from build123d import *

# Parameters (mm, degrees)
F1_DEPTH = 13
F2_R     = 1.5
F4_DEPTH = 4
F5_ANGLE = -90


with BuildPart() as f1:
    # F0 (on Top) → F1 (new body)
    with BuildSketch(Plane.XY):
        Polygon((-40, -45), (-45, 0), (0, 0), (45, 0), (40, -45), (45, -45), (50, 0), (50, 7), (45, 7), (44.8581193677, 7), (-44.8581193677, 7), (-45, 7), (-50, 7), (-50, 0), (-45, -45), align=None)
    extrude(amount=F1_DEPTH)

    # F2
    f2_edges = [f1.edges().sort_by_distance(p)[0] for p in [
        (-42.5, -22.5, 13),
        (0, 0, 13),
        (42.5, -22.5, 13),
        (42.5, -45, 13),
        (47.5, -22.5, 13),
        (50, 3.5, 13),
        (0, 7, 13),
        (-50, 3.5, 13),
        (-47.5, -22.5, 13),
        (-42.5, -45, 13),
        (-42.5, -22.5, 0),
        (0, 0, 0),
        (42.5, -22.5, 0),
        (42.5, -45, 0),
        (47.5, -22.5, 0),
        (50, 3.5, 0),
        (0, 7, 0),
        (-50, 3.5, 0),
        (-47.5, -22.5, 0),
        (-42.5, -45, 0),
        (40, -45, 6.5),
        (45, -45, 6.5),
        (-45, -45, 6.5),
        (-40, -45, 6.5),
        (-45, 0, 6.5),
        (45, 0, 6.5),
        (-50, 7, 6.5),
        (-50, 0, 6.5),
        (50, 0, 6.5),
        (50, 7, 6.5),
    ]]
    fillet(f2_edges, radius=F2_R)

    # F3 (on face) → F4 (cut)
    with BuildSketch(Plane.XZ):
        with BuildLine():
            Line((-14.1421356237, 2.9644660941), (-15.6066017178, 1.5))
            Line((-15.6066017178, 1.5), (15.6066017178, 1.5))
            Line((15.6066017178, 1.5), (14.1421356237, 2.9644660941))
            ThreePointArc((14.1421356237, 2.9644660941), (12.6776695297, 6.5), (14.1421356237, 10.0355339059))
            Line((14.1421356237, 10.0355339059), (15.6066017178, 11.5))
            Line((15.6066017178, 11.5), (-15.6066017178, 11.5))
            Line((-15.6066017178, 11.5), (-14.1421356237, 10.0355339059))
            ThreePointArc((-14.1421356237, 10.0355339059), (-12.6776695297, 6.5), (-14.1421356237, 2.9644660941))
        make_face()
        Polygon((-24.8033008589, 20.6966991411), (-15.6066017178, 11.5), (15.6066017178, 11.5), (24.8033008589, 20.6966991411), (19.5, 26), (14.1966991411, 31.3033008589), (0, 17.1066017178), (-14.1966991411, 31.3033008589), (-19.5, 26), align=None)
        Polygon((-24.8033008589, -7.6966991411), (-19.5, -13), (-14.1966991411, -18.3033008589), (0, -4.1066017178), (14.1966991411, -18.3033008589), (19.5, -13), (24.8033008589, -7.6966991411), (15.6066017178, 1.5), (-15.6066017178, 1.5), align=None)
    extrude(amount=-F4_DEPTH, mode=Mode.SUBTRACT)


with BuildPart() as f1_1:
    # F5: moved
    add(f1.part.rotate(Axis((0, 4, 0), (1, 0, 0)), F5_ANGLE))


solid = f1_1.part
Design review of the part built by this model. Coordinates are the model's own, in mm. A direction names the side the tool comes from. Give positions to 0.01 mm unless a question says otherwise; leave off trailing zeros. Order: outer loops, then holes, each group sorted by start corner. A loop starts at its lowest first (then second) coordinate and runs counter-clockwise, first axis right, second up.
1. Add section A-A, the plane x = -5. State the section outline as (y, z) points, then the cut area to 3 significant figures.
Solution:
outline: (4, -1.5) arc R1.5 ccw to (5.5, -3) - (15.5, -3) arc R1.5 ccw to (17, -1.5) - (17, 0) - (4, 0) - close
area: 38.0 mm2
2. Mouldability with a two-part tool opening along Z and no side actions: class faces 1 (the flat face through (0, 17, -1)), 2 (the flat face through (-42.468, 10.43, 26.792)), 3 (the flat face through (1, 10, -3)) as +Z half, -Z half, draft (parallel to the pull), parting line (faces both ways), or undercut.
Solution:
face 1: draft
face 2: undercut
face 3: -Z half
3. To check wall thickness, follow L1, parallel to Z at x = -17, y = 8.25; L2, parallel to Z at x = 6, y = 8.75; L3, parallel to X at y = 7, z = 1. State the ranges of each line that lie inside material, in increasing order.
Solution:
L1: z = -3 to 4
L2: z = -3 to 0
L3: x = -50 to -14.11, 14.11 to 50
4. Add section C-C, the plane x = 35. State the section outline as (y, z) points.
Solution:
outline: (4, -1.5) arc R1.5 ccw to (5.5, -3) - (15.5, -3) arc R1.5 ccw to (17, -1.5) - (17, 2.5) arc R1.5 ccw to (15.5, 4) - (5.5, 4) arc R1.5 ccw to (4, 2.5) - close
5. Tool access review of faces 4 (the cylindrical face through (42.893, 16.549, 26.839)), 5 (the cylindrical face through (42.893, 4.451, 26.839)), 6 (the flat face through (42.532, 10.43, 26.208)), 7 (the cylindrical face through (12.678, 10.445, 2.028)): name each direction out of +Z, -Z, +X, -X, +Y, -Y from which nothing blocks a thin tool from reaching the whole face with its end or side.
Solution:
face 4: +Y
face 5: -Y
face 6: +Y, -Y
face 7: +Z
6. For pin 1 Ø3 at (x, y) = (34, 8.5) entering from +Z; pin 2 Ø1.5 at (y, z) = (6.5, 41) entering from -X, all flat-tipped, find the tip position at first contact; note any pin that passes through.
Solution:
pin 1: stops at z = 4
pin 2: stops at x = -45.97
7. Add section B-B, the plane y = 11.75. State the section outline as (x, z) points, then the cut area to 3 significant figures.
Solution:
outline: (-50, -1.5) arc R1.5 ccw to (-48.5, -3) - (48.5, -3) arc R1.5 ccw to (50, -1.5) - (50, 3.92) arc R1.5 ccw to (49.99, 4.08) - (45.15, 47.67) arc R1.5 ccw to (43.66, 49) - (41.68, 49) arc R1.5 ccw to (40.19, 47.33) - (44.81, 5.67) arc R1.5 cw to (43.32, 4) - (12.84, 4) - (12.84, 0) - (-12.84, 0) - (-12.84, 4) - (-43.32, 4) arc R1.5 cw to (-44.81, 5.67) - (-40.19, 47.33) arc R1.5 ccw to (-41.68, 49) - (-43.66, 49) arc R1.5 ccw to (-45.15, 47.67) - (-49.99, 4.08) arc R1.5 ccw to (-50, 3.92) - close
area: 1,050 mm2
